Here's the drawing with two shaded views (mm, measured from the low corner). I have some questions. Give positions to 0.01 mm unless a question says otherwise; leave off trailing zeros. Write each loop counter-clockwise with the first axis right and the second up, starting at its lowest first coordinate (ties: lowest second). Pieces come first, ordered by that corner, then holes. Notation, with made-up numbers: (45, 65) -> (103, 65) arc R26 ccw to (103, 93) -> close; hole circle Ø10 at (51.5, -23). An arc over 180 degrees is marked (long way). One line per question, with ' | ' between items.
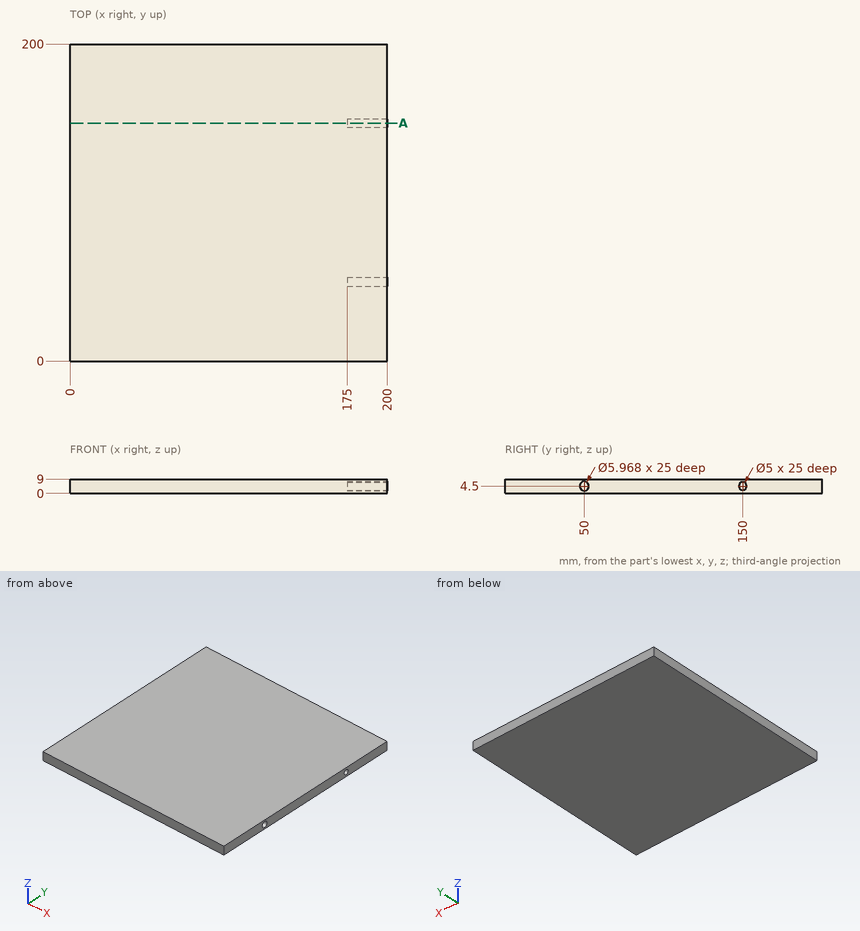
Q1. If I drill on line 1 along Z through (x, y) = (184.25, 150); line 2 along Z through (x, y) = (191.5, 50); line 3 along X through (y, z) = (150, 6.5), over which ranges is the centre line in solid material (lowest first)?
Answer below:
line 1: z = 0 to 2, 7 to 9 | line 2: z = 0 to 1.52, 7.48 to 9 | line 3: x = 0 to 175
Q2. Imagine slicing it at A-A on y = 150. Please give me the cut outline in (x, z).
Answer below:
outline: (0, 0) -> (200, 0) -> (200, 2) -> (175, 2) -> (175, 7) -> (200, 7) -> (200, 9) -> (0, 9) -> close
Q3. Will this pin go through, and if not, where does the flat tip stop? pin 1 (3.5 mm diameter, centred on y = 50, z = 4.5, fed in from +X).
Answer below:
pin 1: stops at x = 175
